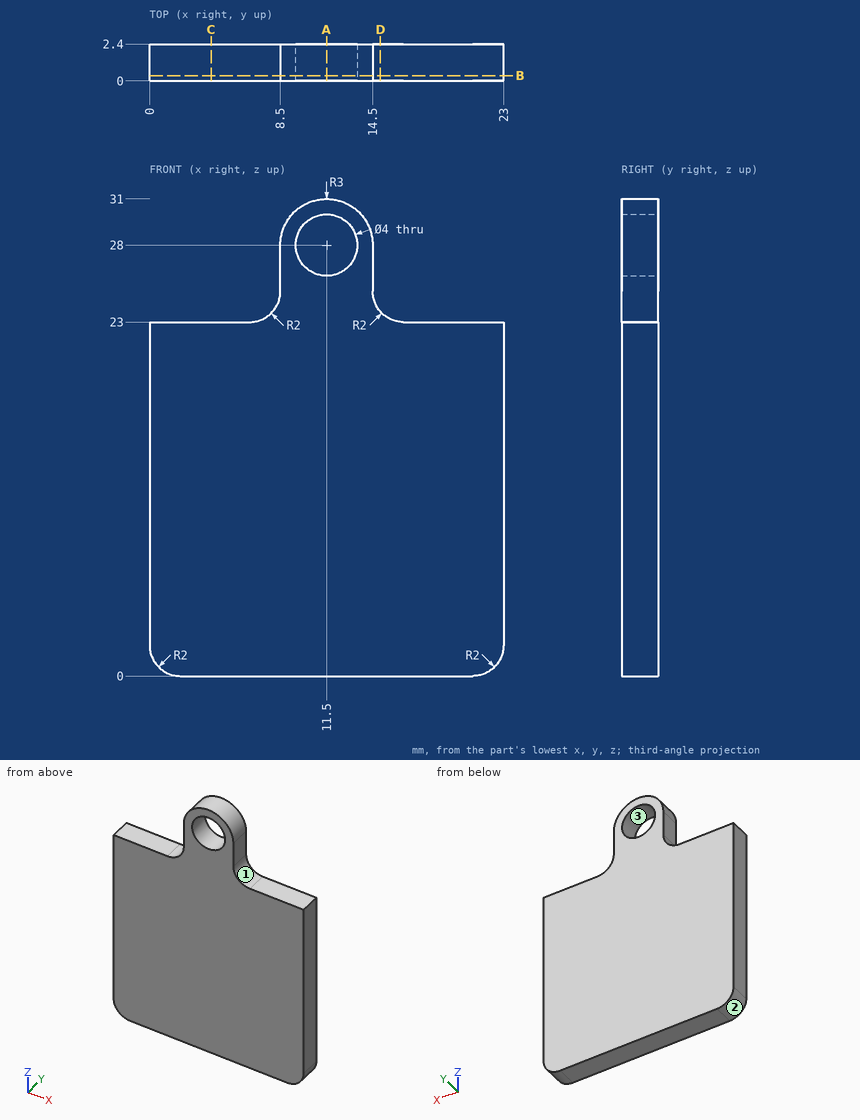
Here's the drawing with two shaded views (mm, measured from the low corner). I have some questions. Coordinates: 2 decimals unless noted, no trailing zeros. Loops run counter-clockwise (first coordinate to the right, second up) from the corner with the lowest first, then second, coordinate; pieces in that order, holes last. Notation, with made-up numbers: M 23,15 L 68,15 A4 ccw 68,21 Z; hole C -17,29 d4. An arc over 180 degrees is marked long. Answer as CSV lines item,"result". Start each with the question number.
1. Thinking about a two-plate mould opening in Z: for the marked faces 1, 2 and 3, which applies, +Z half, -Z half, draft (parallel to the pull), parting line (faces both ways), or undercut?
2. Suppose I cut it at D-D, the plane x = 15. List the corners of the cut face in (y, z) for me.
3. Suppose I cut it at C-C, the plane x = 4. List the corners of the cut face in (y, z) for me, plus the area to 3 significant figures.
4. For pin 1 Ø1.2 at (x, y) = (18, 1) entering from +Z; pin 2 Ø0.7 at (y, z) = (1, 26) entering from -X; pin 3 Ø2.5 at (x, z) = (11.5, 28) entering from -Y, each with a flat end and sliding along its axis, tell me the tip position at first contact or that it passes through.
5. Suppose I cut it at A-A, the plane x = 11.5. List the corners of the cut face in (y, z) for me, plus the area to 3 significant figures.
6. Suppose I cut it at B-B, the plane y = 0.35. List the corners of the cut face in (x, z) for me.
7. If I drill on probe 1 along X at (y, z) = (1, 28); probe 2 along Z at (x, y) = (11.5, 0.55); probe 3 along X at (y, z) = (0.2, 25), over which ranges is the centre line in solid material (lowest first)? Write a range as [from, to].
Output:
1,face 1,"+Z half"
1,face 2,"-Z half"
1,face 3,"undercut"
2,outline,"M 0,0 L 2.4,0 L 2.4,23.68 L 0,23.68 Z"
3,outline,"M 0,0 L 2.4,0 L 2.4,23 L 0,23 Z"
3,area,"55.2 mm^2"
4,pin 1,"stops at z = 23"
4,pin 2,"stops at x = 8.5"
4,pin 3,"passes through"
5,outline,"M 0,0 L 2.4,0 L 2.4,26 L 0,26 Z; M 0,30 L 2.4,30 L 2.4,31 L 0,31 Z"
5,area,"64.8 mm^2"
6,outline,"M 0,2 A2 ccw 2,0 L 21,0 A2 ccw 23,2 L 23,23 L 16.5,23 A2 cw 14.5,25 L 14.5,28 A3 ccw 8.5,28 L 8.5,25 A2 cw 6.5,23 L 0,23 Z; hole C 11.5,28 d4"
7,probe 1,"x = [8.5, 9.5], [13.5, 14.5]"
7,probe 2,"z = [0, 26], [30, 31]"
7,probe 3,"x = [8.5, 14.5]"
